Autodesk Inventor part; units mm, degrees
ref_plane "Plano de trabajo1" through (0, 24.4806, -13.325) normal (0, 0.9239, -0.3827) x (-1, 0, 0)
ref_plane "YZ Plane" through (0, 0, 0) normal (1, 0, 0) x (0, 1, 0)
ref_plane "XZ Plane" through (0, 0, 0) normal (0, 1, 0) x (-1, 0, 0)
sketch "Boceto1" plane through (0, 0, 0) normal (1, 0, 0) x (0, 1, 0)
  line L0 (0, 0) -> (30, 0)
  line L1 (0, 0) -> (30, 0) construction
  line L2 (30, 0) -> (51.2132, -21.2132)
  line L3 (0, 0) -> (0, -12)
  line L4 (0, -12) -> (25.0294, -12)
  line L5 (51.2132, -21.2132) -> (42.7279, -29.6985)
  line L6 (42.7279, -29.6985) -> (25.0294, -12)
  line L7 (0, 0) -> (0, -13.325)
  line L8 (51.2132, -21.2132) -> (41.791, -30.6354)
  line L9 (41.791, -30.6354) -> (24.4806, -13.325)
  line L10 (0, -13.325) -> (24.4806, -13.325)
  line L11 (24.4806, -13.325) -> (24.4806, -12)
  line L12 (24.4806, -13.325) -> (25.4175, -12.3881)
  line L13 (0, 0) -> (30, 0)
  line L14 (51.2132, -21.2132) -> (30, 0)
  point P0 (0, -12)
  dimension "d0" = 30
  dimension "d1" = 0
  dimension "d2" = 30
  dimension "d3" = 135
  dimension "d4" = 12
  dimension "d5" = 12
  dimension "d6" = 13.325
  dimension "d7" = 13.325
revolve "Revolución1" add sketch "Boceto1" angle 360 about axis through (0, 0, 0) along (0, 1, 0) contours L4 L11 L10 L7
revolve "Revolución2" add sketch "Boceto1" angle 360 about axis through (0, 30, 0) along (0, 0.7071, -0.7071) contours L8 L9 L12 L6
ref_plane "Plano de trabajo1" through (0, 24.4806, -13.325) normal (0, 0.9239, -0.3827) x (-1, 0, 0)
sketch "Boceto6" plane through (0, 24.4806, 0) normal (0, 1, 0) x (1, 0, 0)
  circle A0 centre (0, 0) radius 13.325
  circle A1 centre (0, 0) radius 12
  point P0 (0, 13.325)
sketch "Boceto7" plane through (0, 33.9028, -3.9028) normal (0, -0.7071, 0.7071) x (1, 0, 0)
  circle A0 centre (0, 0) radius 13.325
  circle A1 centre (0, 0) radius 12
  point P0 (0, -21.2132)
  point P1 (0, -13.325)
extrude "Extrusión3" add sketch "Boceto6" along normal up to surface surface through (0, 24.4806, -13.325) normal (0, 0.9239, -0.3827)
extrude "Extrusión4" add sketch "Boceto7" along normal up to surface surface through (0, 24.4806, -13.325) normal (0, 0.9239, -0.3827)
fillet "Empalme1" [suppressed]
properties part number "Semicodo"
Build history of the part. All positions in model axes, mm. Coordinates: 2 decimals unless noted, no trailing zeros. Order: outer loops, then holes, each group sorted by start corner. A loop starts at its lowest first (then second) coordinate and runs counter-clockwise, first axis right, second up. Notation, with made-up numbers: (33, -32) - (53, -32) arc R7 ccw to (53, -25) - close; hole circle Ø9 at (-15, -25). An arc over 180 degrees is marked (long way). Put each result on its own line as item: value.
1. Drop flat-ended pins along their axis: P1, Ø6, axis at x = 1, y = 47.5, coming from the +Z side; P2, Ø6, axis at x = -10.5, y = 27, coming from the -Z side; P3, Ø6, axis at y = 21.5, z = -11.5, coming from the +X side; P4, Ø12, axis at y = 50, z = 9, coming from the -X side. Give the stop position or say it passes through.
Answer sheet:
P1: stops at z = 4.3
P2: stops at z = -13.78
P3: stops at x = 10.26
P4: passes through
2. Saw through at B-B (y = 15.5). Write the cut outline in (x, z) (3 decimals).
Answer sheet:
outline: circle Ø26.65 at (0, 0); hole circle Ø24 at (0, 0)
3. Probe line 1 along Z through (x, y) = (0, 11.75) (3 decimals); line 2 along X through (y, z) = (28.5, -9). List the from-to ranges inside material, lowest first. Write a range as [from, to].
Answer sheet:
line 1: z = [-13.325, -12], [12, 13.325]
line 2: x = [-11.06, -9.43], [9.43, 11.06]
4. Pull direction Z, two halves, no side cores. Call faces 1 (the face through (-10.646, 38.521, -16.352)), 2 (the face through (-2, 0, 12)): pulls with the +Z half, pulls with the -Z half, needs draft (parallel to the pull), parting line crosses it, or undercut.
Answer sheet:
face 1: undercut
face 2: needs draft
